Verification items for the finished model (mm, model axes). A direction names the side the tool comes from. Give positions to 0.01 mm unless a question says otherwise; leave off trailing zeros. Write each loop counter-clockwise with the first axis right and the second up, starting at its lowest first coordinate (ties: lowest second). Pieces come first, ordered by that corner, then holes. Notation, with made-up numbers: (-36.5, -11.5) - (13.5, -11.5) arc R22 ccw to (13.5, 25.5) - close; hole circle Ø2 at (46, -16.5). An arc over 180 degrees is marked (long way). Answer as a JSON object with one key per item and string values. Group by question number.
Item 1: Draft check along Y on faces 4 (the face through (347.354, 0.119, -35.807)), 5 (the face through (-5, 9, -15.748)), 6 (the face through (-5, 25.4, -26)). Enter one of: +Y half, -Y half, draft (parallel to the pull), parting line (faces both ways), or undercut.
Item 2: Scan lines: line 1 along Y through (x, z) = (274.5, -28.75); line 2 along Z through (x, y) = (59, -19); line 3 along Z through (x, y) = (165.35, 24.2) (3 decimals). Record each from-to range of solid material in increasing order. Write a range as [from, to].
Item 3: Go/stop test with flat-tipped pins: pin 1 (0.9 mm diameter, centred on y = -3.5, z = -15, fed in from +X); pin 2 (12 mm diameter, centred on y = -12, z = -18, fed in from -X); pin 3 (5 mm diameter, centred on y = -11, z = -16.5, fed in from -X). Record where each tip stops, or that it passes through.
Item 4: Tool access check on faces 1 (the face through (-5, -22.352, -26)), 2 (the face through (5, -16, -38.1)), 3 (the face through (-14.985, 0.66, -36.597)). Record the directions out of +Z, -Z, +X, -X, +Y, -Y that give a thin tool (end or side, any length) a straight path to the whole face; none if there is none.
Item 5: Sectioned sample at A-A, the plane x = 75. Record the boundary of the cut face in (y, z).
```python
from build123d import *

# Parameters (mm, degrees)
BOSS_EXTRUDE1_DEPTH       = 12.7
CUT_EXTRUDE1_DEPTH        = 364.062325917
CUT_EXTRUDE1_DEPTH_BACK   = 364.062325917
SKETCH3_W                 = 19.304
SKETCH3_H                 = 44.704
FILLET1_R                 = 1
WIREHOLE_REACH            = 365.728
MIDDLEHOLE_REACH          = 365.728
SKETCH5_R                 = 15
SPACERHOLESM8_D           = 8.4
WIRE_SLOTS_REACH          = 365.728
PLATE_MOUNTING_REACH      = 367.718
SKETCH14_R                = 4.5
M6X1_0_TAPPED_HOLE1_D     = 5
M6X1_0_TAPPED_HOLE1_DEPTH = 5.588
CUT_EXTRUDE5_DEPTH        = 365.834993524
CUT_EXTRUDE5_DEPTH_BACK   = 365.834993524
SKETCH10_W                = 25.4
SKETCH10_H                = 50.8
POWER_D                   = 16


with BuildPart() as part:
    # Sketch2 → Boss-Extrude1 (new, symmetric)
    with BuildSketch(Plane.XY):
        Polygon((-332.620606325, -25.4), (-361.95, 25.4), (361.95, 25.4), (332.620606325, -25.4), align=None)
    extrude(amount=BOSS_EXTRUDE1_DEPTH, both=True)

    # Sketch3 → Cut-Extrude1 (cut, two sides: drawn at the far end of the back side and taken through both)
    with BuildSketch(Plane(origin=(0, 0, 0), x_dir=(0, 0, -1), z_dir=(1, 0, 0)).offset(-CUT_EXTRUDE1_DEPTH_BACK)):
        Rectangle(SKETCH3_W, SKETCH3_H)
    extrude(amount=CUT_EXTRUDE1_DEPTH + CUT_EXTRUDE1_DEPTH_BACK, mode=Mode.SUBTRACT)

    # Fillet1
    fillet1_edges = [part.edges().sort_by_distance(p)[0] for p in [
        (0, -25.4, 12.7),
        (0, 22.352, -9.652),
        (0, -22.352, -9.652),
        (0, -22.352, 9.652),
        (0, 22.352, 9.652),
        (0, -25.4, -12.7),
        (0, 25.4, -12.7),
        (0, 25.4, 12.7),
    ]]
    fillet(fillet1_edges, radius=FILLET1_R)

    # Sketch4 → WireHole (cut, up to next)
    with BuildSketch(Plane(origin=(0, 0, -12.7), x_dir=(-1, 0, 0), z_dir=(0, 0, -1)), mode=Mode.PRIVATE) as wirehole_sk1:
        with BuildLine():
            Line((-7, 0), (-7, -10))
            ThreePointArc((-7, -10), (0, -17), (7, -10))
            Line((7, -10), (7, 0))
            ThreePointArc((7, 0), (0, 7), (-7, 0))
        make_face()
    wirehole_tool1 = extrude(wirehole_sk1.sketch, amount=-WIREHOLE_REACH, mode=Mode.PRIVATE) & part.part
    add(wirehole_tool1.solids().sort_by_distance((0, -5, -12.7))[0], mode=Mode.SUBTRACT)

    # Sketch5 → MiddleHole (cut, up to next)
    with BuildSketch(Plane.XY.offset(12.7), mode=Mode.PRIVATE) as middlehole_sk1:
        Circle(SKETCH5_R)
    middlehole_tool1 = extrude(middlehole_sk1.sketch, amount=-MIDDLEHOLE_REACH, mode=Mode.PRIVATE) & part.part
    add(middlehole_tool1.solids().sort_by_distance((0, 0, 12.7))[0], mode=Mode.SUBTRACT)

    # SpacerHolesM8 (through all)
    with Locations(Plane.XY.offset(12.7)):
        with Locations((-25.5, 0), (25.5, 0)):
            Hole(SPACERHOLESM8_D / 2)

    # Sketch9 → Wire Slots (cut, up to next)
    with BuildSketch(Plane(origin=(0, 0, -12.7), x_dir=(-1, 0, 0), z_dir=(0, 0, -1)), mode=Mode.PRIVATE) as wire_slots_sk1:
        with BuildLine():
            Line((-222.25, 7.14375), (-215.9, 7.14375))
            ThreePointArc((-215.9, 7.14375), (-208.75625, 0), (-215.9, -7.14375))
            Line((-215.9, -7.14375), (-222.25, -7.14375))
            ThreePointArc((-222.25, -7.14375), (-229.39375, 0), (-222.25, 7.14375))
        make_face()
    wire_slots_tool1 = extrude(wire_slots_sk1.sketch, amount=-WIRE_SLOTS_REACH, mode=Mode.PRIVATE) & part.part
    # Sketch9 → Wire Slots (cut, up to next)
    with BuildSketch(Plane(origin=(0, 0, -12.7), x_dir=(-1, 0, 0), z_dir=(0, 0, -1)), mode=Mode.PRIVATE) as wire_slots_sk2:
        with BuildLine():
            Line((222.25, 7.14375), (215.9, 7.14375))
            ThreePointArc((215.9, 7.14375), (208.75625, 0), (215.9, -7.14375))
            Line((215.9, -7.14375), (222.25, -7.14375))
            ThreePointArc((222.25, -7.14375), (229.39375, 0), (222.25, 7.14375))
        make_face()
    wire_slots_tool2 = extrude(wire_slots_sk2.sketch, amount=-WIRE_SLOTS_REACH, mode=Mode.PRIVATE) & part.part
    add(wire_slots_tool1.solids().sort_by_distance((219.075, 0, -12.7))[0], mode=Mode.SUBTRACT)
    add(wire_slots_tool2.solids().sort_by_distance((-219.075, 0, -12.7))[0], mode=Mode.SUBTRACT)

    # Sketch14 → Plate Mounting (cut, up to next)
    with BuildSketch(Plane(origin=(0, 25.4, 0), x_dir=(1, 0, 0), z_dir=(0, 1, 0)), mode=Mode.PRIVATE) as plate_mounting_sk1:
        with Locations(Location((-165.35, 1.475, 0), (0, 0, 180))):
            Circle(SKETCH14_R)
    plate_mounting_tool1 = extrude(plate_mounting_sk1.sketch, amount=-PLATE_MOUNTING_REACH, mode=Mode.PRIVATE) & part.part
    # Sketch14 → Plate Mounting (cut, up to next)
    with BuildSketch(Plane(origin=(0, 25.4, 0), x_dir=(1, 0, 0), z_dir=(0, 1, 0)), mode=Mode.PRIVATE) as plate_mounting_sk2:
        with Locations(Location((-292.35, 1.475, 0), (0, 0, 180))):
            Circle(SKETCH14_R)
    plate_mounting_tool2 = extrude(plate_mounting_sk2.sketch, amount=-PLATE_MOUNTING_REACH, mode=Mode.PRIVATE) & part.part
    # Sketch14 → Plate Mounting (cut, up to next)
    with BuildSketch(Plane(origin=(0, 25.4, 0), x_dir=(1, 0, 0), z_dir=(0, 1, 0)), mode=Mode.PRIVATE) as plate_mounting_sk3:
        with Locations(Location((292.35, 1.475, 0), (0, 0, 180))):
            Circle(SKETCH14_R)
    plate_mounting_tool3 = extrude(plate_mounting_sk3.sketch, amount=-PLATE_MOUNTING_REACH, mode=Mode.PRIVATE) & part.part
    # Sketch14 → Plate Mounting (cut, up to next)
    with BuildSketch(Plane(origin=(0, 25.4, 0), x_dir=(1, 0, 0), z_dir=(0, 1, 0)), mode=Mode.PRIVATE) as plate_mounting_sk4:
        with Locations(Location((165.35, 1.475, 0), (0, 0, 180))):
            Circle(SKETCH14_R)
    plate_mounting_tool4 = extrude(plate_mounting_sk4.sketch, amount=-PLATE_MOUNTING_REACH, mode=Mode.PRIVATE) & part.part
    add(plate_mounting_tool1.solids().sort_by_distance((-165.35, 25.4, -1.475))[0], mode=Mode.SUBTRACT)
    add(plate_mounting_tool2.solids().sort_by_distance((-292.35, 25.4, -1.475))[0], mode=Mode.SUBTRACT)
    add(plate_mounting_tool3.solids().sort_by_distance((292.35, 25.4, -1.475))[0], mode=Mode.SUBTRACT)
    add(plate_mounting_tool4.solids().sort_by_distance((165.35, 25.4, -1.475))[0], mode=Mode.SUBTRACT)

    # M6x1.0 Tapped Hole1
    with Locations(Plane(origin=(0, 0, 15.24), x_dir=(-1, 0, 0), z_dir=(0, 0, 1))):
        with Locations((-330.2, 0), (330.2, 0)):
            Hole(M6X1_0_TAPPED_HOLE1_D / 2, depth=M6X1_0_TAPPED_HOLE1_DEPTH)


with BuildPart() as body_2:
    # Mirror1: mirrored copy
    add(part.part.mirror(Plane(origin=(0, 0, -12.7), x_dir=(1, 0, 0), z_dir=(0, 0, -1))))

    # Power (through all)
    with Locations(Plane(origin=(0, 0, -38.1), x_dir=(-1, 0, 0), z_dir=(0, 0, -1))):
        with Locations((254, 0)):
            Hole(POWER_D / 2)


with BuildPart() as part_1:
    add(part.part)

    # Sketch10 → Cut-Extrude5 (cut, two sides: drawn at the far end of the back side and taken through both)
    with BuildSketch(Plane(origin=(0, 0, 0), x_dir=(0, 0, -1), z_dir=(1, 0, 0)).offset(-CUT_EXTRUDE5_DEPTH_BACK)):
        Rectangle(SKETCH10_W, SKETCH10_H)
    extrude(amount=CUT_EXTRUDE5_DEPTH + CUT_EXTRUDE5_DEPTH_BACK, mode=Mode.SUBTRACT)


solid = body_2.part
```
Geometry check:
{
 "1": {"face 4": "-Y half", "face 5": "undercut", "face 6": "+Y half"},
 "2": {"line 1": "[-25.4, -22.35], [22.35, 25.4]", "line 2": "[-38.1, -35.05], [-15.75, -12.7]", "line 3": "[-38.1, -28.425], [-19.425, -12.7]"},
 "3": {"pin 1": "x = 345.52", "pin 2": "x = -343.57", "pin 3": "x = -342.31"},
 "4": {"face 1": "+X, -X", "face 2": "-Z, +X, -X, +Y, -Y", "face 3": "-Z"},
 "5": {"outline": "(-25.4, -37.1) arc R1 ccw to (-24.4, -38.1) - (24.4, -38.1) arc R1 ccw to (25.4, -37.1) - (25.4, -13.7) arc R1 ccw to (24.4, -12.7) - (-24.4, -12.7) arc R1 ccw to (-25.4, -13.7) - close; hole (-22.35, -34.05) arc R1 ccw to (-21.35, -35.05) - (21.35, -35.05) arc R1 ccw to (22.35, -34.05) - (22.35, -16.75) arc R1 ccw to (21.35, -15.75) - (-21.35, -15.75) arc R1 ccw to (-22.35, -16.75) - close"}
}
